Model file for the job. Use its own axes, mm. Face numbers are marked on the shaded views. A direction names the side the tool comes from. Coordinates: 2 decimals unless noted, no trailing zeros. Loops run counter-clockwise (first coordinate to the right, second up) from the corner with the lowest first, then second, coordinate; pieces in that order, holes last. Notation, with made-up numbers: M 56,61 L 101,61 A13 ccw 101,68 Z; hole C -16.5,-27.75 d1. An arc over 180 degrees is marked long. One line per question, with ' | ' between items. Start each with the question number.
Autodesk Inventor part; units mm, degrees
ref_plane "YZ Plane" through (0, 0, 0) normal (1, 0, 0) x (0, 1, 0)
ref_plane "XZ Plane" through (0, 0, 0) normal (0, 1, 0) x (-1, 0, 0)
ref_plane "XY Plane" through (0, 0, 0) normal (0, 0, 1) x (1, 0, 0)
sketch "Boceto1" plane through (0, 0, 0) normal (0, 1, 0) x (-1, 0, 0)
  line L0 (10.05, 40.05) -> (-10.05, 40.05)
  line L1 (-10.05, 40.05) -> (-10.05, -40.05)
  line L2 (-10.05, -40.05) -> (10.05, -40.05)
  line L3 (10.05, -40.05) -> (10.05, 40.05)
  line L4 (10.05, 40.05) -> (-10.05, -40.05) construction
  line L5 (-10.05, 40.05) -> (10.05, -40.05) construction
  line L6 (12.05, 42.05) -> (-12.05, 42.05)
  line L7 (-12.05, 42.05) -> (-12.05, -42.05)
  line L8 (-12.05, -42.05) -> (12.05, -42.05)
  line L9 (12.05, -42.05) -> (12.05, 42.05)
  point P0 (0, 0)
  dimension "d0" = 20.1
  dimension "d1" = 80.1
  dimension "d2" = 2
extrude "Extrusión1" add sketch "Boceto1" along normal blind 2 contours L3 L2 L1 L0 | L9 L8 L7 L6
sketch "Boceto2" plane through (0, 2, 0) normal (0, 1, 0) x (1, 0, 0)
  line L0 (12.05, -42.05) -> (12.05, 42.05)
  line L1 (-12.05, -42.05) -> (12.05, -42.05)
  line L2 (12.05, -42.05) -> (12.05, 42.05)
  line L3 (-12.05, 42.05) -> (-12.05, -42.05)
  line L4 (-12.05, -42.05) -> (12.05, 42.05) construction
  line L5 (12.05, -42.05) -> (-12.05, 42.05) construction
  line L6 (-10.05, -40.05) -> (10.05, -40.05)
  line L7 (10.05, -40.05) -> (10.05, 40.15)
  line L8 (-10.05, 40.05) -> (-10.05, -40.05)
  line L9 (-10.05, 40.05) -> (-10.05, 42.05)
  line L10 (10.05, 40.15) -> (10.05, 42.05)
  line L11 (12.05, 42.05) -> (-12.05, 42.05)
  line L12 (12.05, 42.05) -> (10.05, 42.05)
  line L13 (-12.05, 42.05) -> (-10.05, 42.05)
  line L14 (-12.05, 42.05) -> (-12.05, -42.05)
  line L15 (-12.05, 24.05) -> (-10.05, 24.05)
  line L16 (-12.05, -27.6873) -> (-10.05, -27.6873)
  line L17 (-10.05, -27.6873) -> (-10.05, -12.6873)
  line L18 (-10.05, -12.6873) -> (-12.05, -12.6873)
  line L19 (-12.05, -12.6873) -> (-12.05, -27.6873)
  line L20 (-8.05, -40.05) -> (-8.05, -42.05)
  line L21 (-12.05, -42.05) -> (12.05, -42.05)
  line L22 (8.05, -40.05) -> (8.05, -42.05)
  point P0 (0, 0)
  point P1 (8.05, -41.05)
  point P2 (-12.05, 24.05)
  dimension "d5" = 2
  dimension "d8" = 18
  dimension "d9" = 15
  dimension "d10" = 12.3627
  dimension "d11" = 2
  dimension "d12" = 2
  dimension "d13" = 4
  dimension "d14" = 4
extrude "Extrusión2" add sketch "Boceto2" along normal blind 7 contours L1 L22 L6 L7 L10 L11 L0 | L1 L3 L16 L8 L6 L20 | L3 L18 L8 L16 | L8 L18 L3 L15
sketch "Boceto5" plane through (0, 0, 0) normal (0, 1, 0) x (-1, 0, 0)
  line L0 (-12.05, -30.296) -> (-26.35, -30.296)
  line L1 (-26.35, -30.296) -> (-26.35, 8.704)
  line L2 (-26.35, 8.704) -> (-12.05, 8.704)
  line L3 (-12.05, 8.704) -> (-12.05, -30.296)
  line L4 (-12.05, -30.296) -> (-26.35, 8.704) construction
  line L5 (-26.35, -30.296) -> (-12.05, 8.704) construction
  line L6 (-12.05, 42.05) -> (-12.05, -42.05)
  line L7 (-28.35, -32.296) -> (-10.05, -32.296)
  line L8 (-10.05, -32.296) -> (-10.05, 10.704)
  line L9 (-10.05, 10.704) -> (-28.35, 10.704)
  line L10 (-28.35, 10.704) -> (-28.35, -32.296)
  point P0 (0, 0)
  point P1 (-19.2, -10.796)
  point P2 (-12.05, 10.704)
  point P3 (-12.05, -32.296)
  dimension "d25" = 14.3
  dimension "d26" = 39
  dimension "d27" = 0
  dimension "d28" = 2
extrude "Extrusión5" add sketch "Boceto5" along normal blind 14 contours L6 L7 L10 L9 L2 L1 L0 | L0 L1 L2 L3
sketch "Boceto6" plane through (0, 14, 0) normal (0, 1, 0) x (1, 0, 0)
  line L0 (28.35, 32.296) -> (12.05, 32.296)
  line L1 (20.2, 32.296) -> (20.2, 4.5557)
  line L2 (14.05, 30.296) -> (26.35, 30.296)
  line L3 (26.35, 30.296) -> (26.35, -8.704)
  line L4 (26.35, -8.704) -> (14.05, -8.704)
  line L5 (14.05, 30.296) -> (26.35, -8.704) construction
  line L6 (26.35, 30.296) -> (14.05, -8.704) construction
  line L7 (28.35, -10.704) -> (28.35, 32.296)
  line L8 (12.05, -10.704) -> (28.35, -10.704)
  line L9 (14.05, -8.704) -> (12.05, -8.704)
  line L10 (12.05, -8.704) -> (12.05, 30.296)
  line L11 (12.05, 32.296) -> (12.05, -10.704)
  line L12 (14.05, 30.296) -> (12.05, 30.296)
  line L13 (28.35, -10.704) -> (28.35, 32.296)
  line L14 (28.35, -8.704) -> (28.35, -10.704)
  line L15 (12.05, -10.704) -> (28.35, -10.704)
  line L16 (15.2, -8.704) -> (25.2, -8.704)
  line L17 (25.2, -8.704) -> (25.2, -10.704)
  line L18 (25.2, -10.704) -> (15.2, -10.704)
  line L19 (15.2, -10.704) -> (15.2, -8.704)
  line L20 (15.2, -8.704) -> (25.2, -10.704) construction
  line L21 (25.2, -8.704) -> (15.2, -10.704) construction
  line L22 (26.35, 30.296) -> (26.35, 32.296)
  point P0 (0, 0)
  point P1 (20.2, 10.796)
  point P2 (20.2, -8.704)
  point P3 (20.2, -9.704)
  point P4 (15.2, -8.704)
  point P5 (15.2, -10.704)
  point P6 (25.2, -10.704)
  dimension "d31" = 2
  dimension "d32" = 2
  dimension "d33" = 2
  dimension "d34" = 10
extrude "Extrusión6" cut sketch "Boceto6" against normal blind 12 contours L22 L2 L1 L0 | L1 L2 L12 L11 L0 | L3 L4 L9 L10 L12 L2 | L8 L19 L4 L17
sketch "Boceto8" plane through (0, 0, 0) normal (0, 1, 0) x (-1, 0, 0)
  line L0 (12.05, 27.05) -> (18.05, 27.05)
  line L1 (18.05, 27.05) -> (18.05, 3.05)
  line L2 (18.05, 3.05) -> (12.05, 3.05)
  line L3 (12.05, 3.05) -> (12.05, 27.05)
  line L4 (12.05, -24.05) -> (12.05, 42.05)
  line L5 (8.05, 42.05) -> (-8.05, 42.05)
  point P0 (0, 0)
  dimension "d44" = 6
  dimension "d45" = 24
  dimension "d46" = 0
  dimension "d47" = 15
extrude "Extrusión8" add sketch "Boceto8" along normal blind 25
sketch "Boceto10" plane through (0, 9, 0) normal (0, 1, 0) x (1, 0, 0)
  line L0 (-12.05, -3.05) -> (-18.05, -3.05)
  line L1 (-10.05, -40.05) -> (-10.05, 24.05)
  line L2 (-12.05, -3.05) -> (-10.05, -3.05)
  line L3 (-10.05, -3.05) -> (-10.05, -27.05)
  line L4 (-10.05, -27.05) -> (-12.05, -27.05)
  line L5 (-12.05, -27.05) -> (-12.05, -3.05)
  line L6 (-18.05, -27.05) -> (-12.05, -27.05)
  point P0 (0, 0)
  point P1 (-10.05, -3.05)
  point P2 (-11.05, -27.05)
  dimension "d65" = 0
extrude "Extrusión10" add sketch "Boceto10" along normal blind 16
sketch "Boceto11" plane through (-18.05, 0, 3.05) normal (-1, 0, 0) x (0, 0, 1)
  line L0 (4.5, 21.5) -> (19.5, 21.5)
  line L1 (19.5, 21.5) -> (19.5, 12.5)
  line L2 (19.5, 12.5) -> (4.5, 12.5)
  line L3 (4.5, 12.5) -> (4.5, 21.5)
  line L4 (4.5, 21.5) -> (19.5, 12.5) construction
  line L5 (19.5, 21.5) -> (4.5, 12.5) construction
  line L6 (0, 25) -> (24, 25)
  line L7 (-27.1, 9) -> (0, 9)
  line L8 (24, 25) -> (0, 25)
  line L9 (12, 25) -> (12, 17)
  point P0 (-3.05, 0)
  dimension "d59" = 15
  dimension "d60" = 9
  dimension "d61" = 3.5
  dimension "d62" = 3.5
  dimension "d66" = 0
extrude "Extrusión11" cut sketch "Boceto11" against normal blind 8
sketch "Boceto13" plane through (0, 0, 0) normal (0, 1, 0) x (-1, 0, 0)
  line L0 (28.35, -42.05) -> (-28.35, -42.05)
  line L1 (-28.35, -42.05) -> (-28.35, 42.05)
  line L2 (-28.35, 42.05) -> (28.35, 42.05)
  line L3 (28.35, 42.05) -> (28.35, -42.05)
  line L4 (28.35, -42.05) -> (-28.35, 42.05) construction
  line L5 (-28.35, -42.05) -> (28.35, 42.05) construction
  line L6 (-28.35, 10.704) -> (-28.35, -32.296)
  line L7 (-8.05, 42.05) -> (-12.05, 42.05)
  circle A0 centre (23.35, -37.05) radius 1.75
  line L8 (-12.05, -42.05) -> (12.05, -42.05)
  line L9 (0, -42.05) -> (0, -48.6371)
  line L10 (28.35, 0) -> (35.954, 0)
  circle A1 centre (-23.35, -37.05) radius 1.75
  circle A2 centre (23.35, 37.05) radius 1.75
  circle A3 centre (-23.35, 37.05) radius 1.75
  point P0 (0, 0)
  dimension "d67" = 0
  dimension "d68" = 0
  dimension "d72" = 3.5
  dimension "d73" = 5
  dimension "d74" = 5
extrude "Extrusión12" add sketch "Boceto13" along normal blind 2
properties part number "light_indicator"
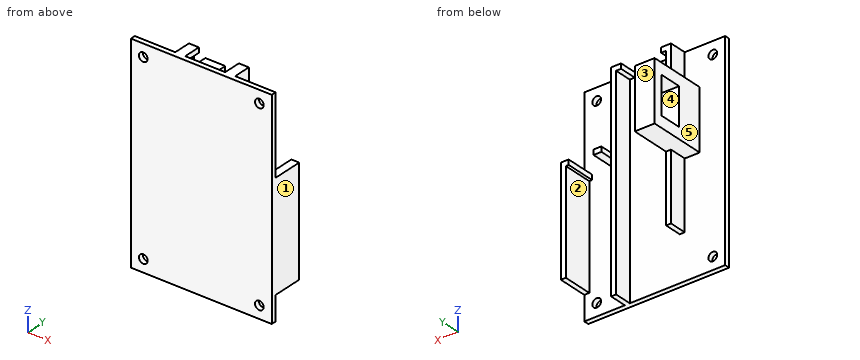
(1) Band-saw the part on C-C on z = 37.05. Write the cut outline in (x, y).
(2) Two-plate mould, pull along Y, no slides. Class the marked faces 3, 4 and 5: pulls with the +Y half, pulls with the -Y half, needs draft (parallel to the pull), parting line crosses it, or undercut.
(3) Drill centre lines: line 1 (X direction, y = 3.25, z = -17.5); line 2 (Z direction, x = -23.35, y = 0.75); line 3 (Y direction, x = -26, z = -16.5). Where is each one in solid material? Low to high. Write a range as [from, to].
(4) 3-axis set-ups, long thin cutter, end or side, ignore diameter. For the marked faces 1 and 2: which of +Z, -Z, +X, -X, +Y, -Y reach the whole face in a straight line?
(5) Band-saw the part on A-A on y = 19. Write the cut outline in (x, z), then the cut area to 3 significant figures.
(6) Band-saw the part on D-D on x = 23.35. Write the cut outline in (y, z), then the cut area to 3 significant figures.
(7) Pin check, flat tips, straight feed: P1, Ø13, axis at x = 16, z = -7.5, coming from the +Y side; P2, Ø2, axis at x = -1, z = 16.5, coming from the +Y side; P3, Ø3.5, axis at y = 7, z = 2.5, coming from the -X side. Stop position of each tip, or through.
(8) Band-saw the part on B-B on z = 14. Write the cut outline in (x, y).
Computed values:
1) outline: M -28.35,0 L -25.1,0 L -25.1,2 L -28.35,2 Z; M -21.6,0 L 21.6,0 L 21.6,2 L 12.05,2 L 12.05,9 L 10.05,9 L 10.05,2 L -10.05,2 L -10.05,9 L -12.05,9 L -12.05,2 L -21.6,2 Z; M 25.1,0 L 28.35,0 L 28.35,2 L 25.1,2 Z
2) face 3: pulls with the +Y half | face 4: undercut | face 5: needs draft
3) line 1: [-12.05, -10.05], [10.05, 12.05], [26.35, 28.35] | line 2: [-42.05, -38.8], [-35.3, 35.3], [38.8, 42.05] | line 3: [0, 2]
4) face 1: +Z, -Z, +X, +Y, -Y | face 2: -Z, +Y
5) outline: M -18.05,3.05 L -10.05,3.05 L -10.05,7.55 L -18.05,7.55 Z; M -18.05,22.55 L -10.05,22.55 L -10.05,27.05 L -18.05,27.05 Z | area: 72.0 mm^2
6) outline: M 0,-42.05 L 2,-42.05 L 2,-38.8 L 0,-38.8 Z; M 0,-35.3 L 2,-35.3 L 2,35.3 L 0,35.3 Z; M 0,38.8 L 2,38.8 L 2,42.05 L 0,42.05 Z | area: 154 mm^2
7) P1: y = 9 | P2: y = 2 | P3: x = -18.05
8) outline: M -28.35,0 L 28.35,0 L 28.35,2 L 12.05,2 L 12.05,9 L 10.05,9 L 10.05,2 L -10.05,2 L -10.05,12.5 L -18.05,12.5 L -18.05,2 L -28.35,2 Z; M -18.05,21.5 L -10.05,21.5 L -10.05,25 L -18.05,25 Z
